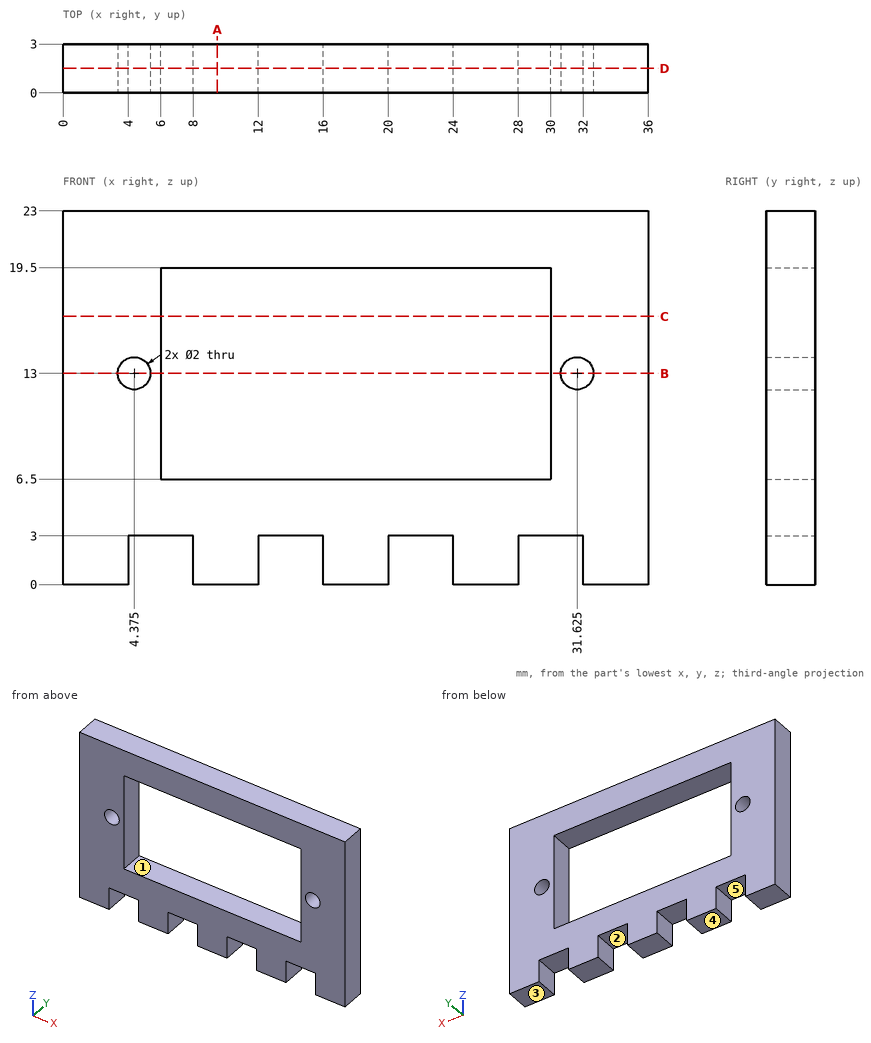
Study the drawing (mm; zero at the part's minimum x, y, z) and answer. A direction names the side the tool comes from. Coordinates: 2 decimals unless noted, no trailing zeros. Loops run counter-clockwise (first coordinate to the right, second up) from the corner with the lowest first, then second, coordinate; pieces in that order, holes last. Notation, with made-up numbers: M 4.5,78 L 8.5,78 A27 cw 8.5,106 Z; hole C 1,-18 d8. An arc over 180 degrees is marked long. Answer in a Markdown table with one row per item. Add a question column.
1. Find section B-B, the plane z = 13. Write down the section's boundary in (x, y) (3 decimals).
2. A tool of negligible diameter and unlimited length cuts with its end or side. For the marked faces 1, 2 and 3, from which of +Z, -Z, +X, -X, +Y, -Y can it reach the whole face along a straight path? Write none if from no direction.
3. Find section D-D, the plane y = 1.5. Write down the section's boundary in (x, z) (3 decimals), then the cut area to 3 significant figures.
4. Consider L1, parallel to X at y = 0.25, z = 2.75; L2, parallel to X at y = 2.2, z = 13 (3 decimals); L3, parallel to Z at x = 25, y = 2.4. Determine where each line is inside the solid, lowest interval first.
5. Find section A-A, the plane x = 9.5. Write down the section's boundary in (y, z), then the cut area to 3 significant figures.
6. A flat-ended cylindrical pin translates along its axis: P1, Ø1.5, axis at x = 13.5, y = 1.5, coming from the -Z side. Find the tip coordinate at first contact, or state that the pin passes through.
7. The mould has two halves that part along X. Classify the marked faces 4 and 5: pulls with the +X half, pulls with the -X half, needs draft (parallel to the pull), parting line crosses it, or undercut.
8. Find section C-C, the plane z = 16.5. Write down the section's boundary in (x, y).
Reported:
| question | item | result |
|---|---|---|
| 1 | outline | M 0,0 L 3.375,0 L 3.375,3 L 0,3 Z; M 5.375,0 L 6,0 L 6,3 L 5.375,3 Z; M 30,0 L 30.625,0 L 30.625,3 L 30,3 Z; M 32.625,0 L 36,0 L 36,3 L 32.625,3 Z |
| 2 | face 1 | +Y, -Y |
| 2 | face 2 | -Z, +Y, -Y |
| 2 | face 3 | -Z, +X, -X, +Y, -Y |
| 3 | outline | M 0,0 L 4,0 L 4,3 L 8,3 L 8,0 L 12,0 L 12,3 L 16,3 L 16,0 L 20,0 L 20,3 L 24,3 L 24,0 L 28,0 L 28,3 L 32,3 L 32,0 L 36,0 L 36,23 L 0,23 Z; hole C 4.375,13 d2; hole M 6,6.5 L 30,6.5 L 30,19.5 L 6,19.5 Z; hole C 31.625,13 d2 |
| 3 | area | 462 mm^2 |
| 4 | L1 | x = 0 to 4, 8 to 12, 16 to 20, 24 to 28, 32 to 36 |
| 4 | L2 | x = 0 to 3.375, 5.375 to 6, 30 to 30.625, 32.625 to 36 |
| 4 | L3 | z = 0 to 6.5, 19.5 to 23 |
| 5 | outline | M 0,0 L 3,0 L 3,6.5 L 0,6.5 Z; M 0,19.5 L 3,19.5 L 3,23 L 0,23 Z |
| 5 | area | 30.0 mm^2 |
| 6 | P1 | stops at z = 3 |
| 7 | face 4 | needs draft |
| 7 | face 5 | undercut |
| 8 | outline | M 0,0 L 6,0 L 6,3 L 0,3 Z; M 30,0 L 36,0 L 36,3 L 30,3 Z |
